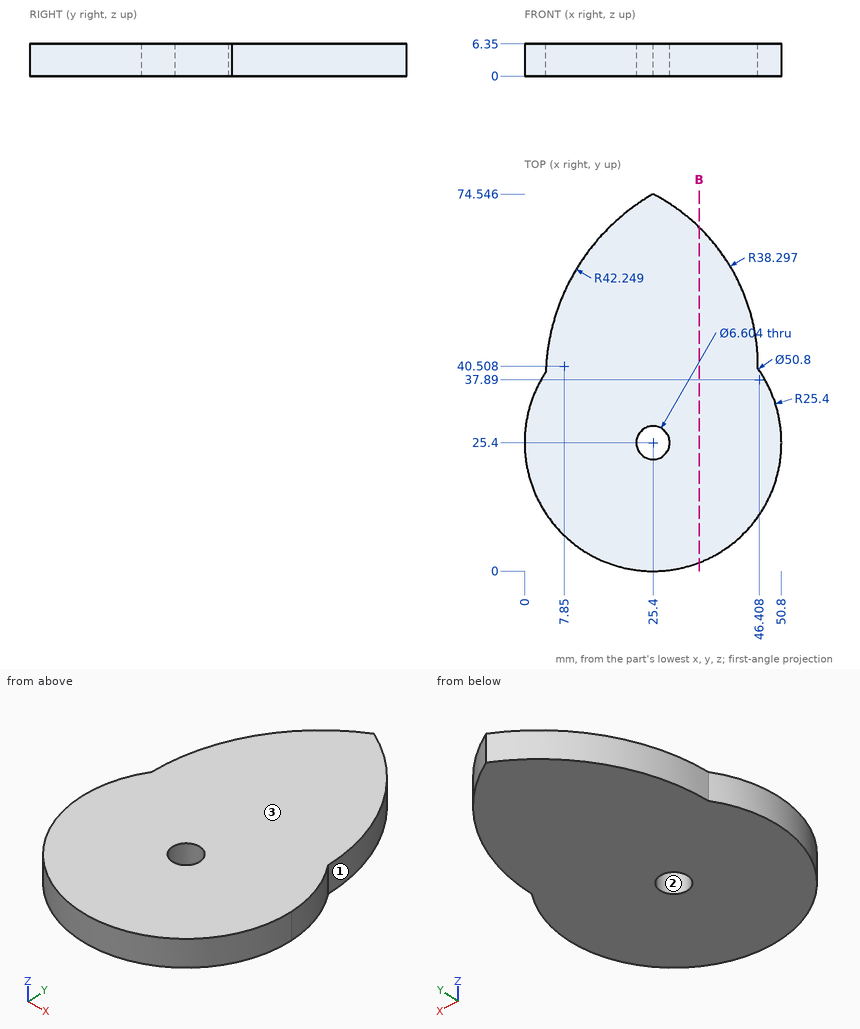
Answer from the drawing. Dimensions are ordinates in mm from the lowest x, y and z of the part. Give positions to 0.01 mm unless a question says otherwise; leave off trailing zeros. Loops run counter-clockwise (first coordinate to the right, second up) from the corner with the lowest first, then second, coordinate; pieces in that order, holes last.
Item 1: A cutting plane is placed at B-B (x = 34.5). Give the vertices of the cut face in (y, z).
Derived:
outline: (1.69, 0) - (68.01, 0) - (68.01, 6.35) - (1.69, 6.35) - close
Item 2: Determine the mould class of the marked faces 1, 2 and 3 for opening direction X: +X half, -X half, draft (parallel to the pull), parting line (faces both ways), or undercut.
Derived:
face 1: +X half
face 2: undercut
face 3: draft
Item 3: Find the intervals of material crossed by line 1 along Y through (x, z) = (15.5, 4.75) (1 decimal); line 2 along Y through (x, z) = (24.5, 3) (1 decimal); line 3 along X through (y, z) = (48, 0.5) (1 decimal), in increasing order.
Derived:
line 1: y = 2 to 66.7
line 2: y = 0 to 22.2, 28.6 to 74
line 3: x = 5.4 to 45.4
